Geometry: see drawing. Coordinates: mm, zero at the bounding-box minimum. A direction names the side the tool comes from. Coordinates: 2 decimals unless noted, no trailing zeros. Loops run counter-clockwise (first coordinate to the right, second up) from the corner with the lowest first, then second, coordinate; pieces in that order, holes last. Notation, with made-up numbers: (72, -11) - (121, -11) arc R32 ccw to (121, 15) - close; hole circle Ø1 at (50.25, 5). An arc over 180 degrees is marked (long way). Answer in a Markdown table with one row per item.
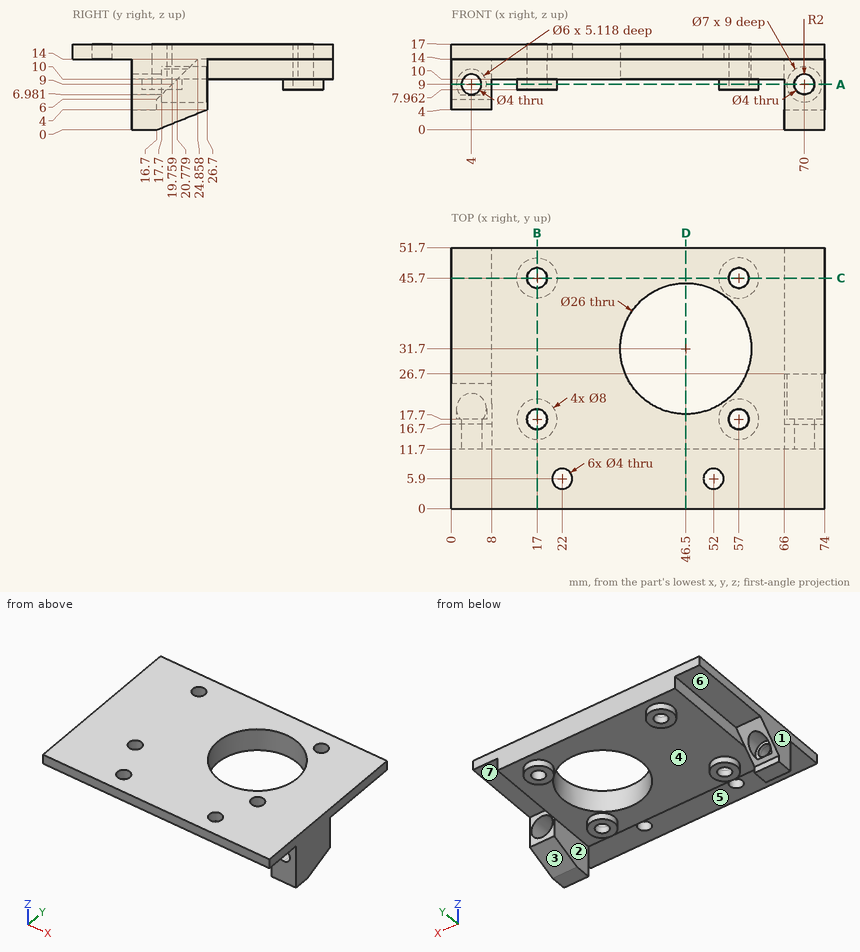
(1) Cut plane D-D on x = 46.5. Output: boundary loops of the cut face in (y, z).
Verdict:
| item | result |
|---|---|
| outline | (0, 14) - (11.7, 14) - (11.7, 10) - (18.7, 10) - (18.7, 17) - (0, 17) - close; (44.7, 10) - (51.7, 10) - (51.7, 17) - (44.7, 17) - close |
(2) Access query for the marked faces 5, 6 and 7. Directions: +Z, -Z, +X, -X, +Y, -Y. A direction counts if a zero-diameter tool reaches every point of the face in a straight line with its end or side. Return the directions, or none.
Verdict:
| item | result |
|---|---|
| face 5 | -Z, +X, -X, -Y |
| face 6 | -Z, -X, +Y |
| face 7 | -Z, +X, +Y |
(3) Cut plane B-B on x = 17. Output: boundary loops of the cut face in (y, z).
Verdict:
| item | result |
|---|---|
| outline | (0, 14) - (11.7, 14) - (11.7, 10) - (13.7, 10) - (13.7, 7.96) - (15.7, 7.96) - (15.7, 17) - (0, 17) - close; (19.7, 7.96) - (21.7, 7.96) - (21.7, 10) - (41.7, 10) - (41.7, 7.96) - (43.7, 7.96) - (43.7, 17) - (19.7, 17) - close; (47.7, 7.96) - (49.7, 7.96) - (49.7, 10) - (51.7, 10) - (51.7, 17) - (47.7, 17) - close |
(4) Pull-direction query (X, two-part tool) for the marked faces 1, 2, 3 and 4; classes: pulls with the +X half, pulls with the -X half, needs draft (parallel to the pull), parting line crosses it, or undercut.
Verdict:
| item | result |
|---|---|
| face 1 | pulls with the -X half |
| face 2 | undercut |
| face 3 | needs draft |
| face 4 | undercut |
(5) First-contact query: pin 1 Ø2 at (y, z) = (27.5, 10) entering from -X; pin 2 Ø3 at (x, z) = (12.5, 11) entering from -Y; pin 3 Ø4.5 at (x, y) = (22, 5.9) entering from -Z. Flat tips, straight axial feed; report the tip coordinate or a pass-through.
Verdict:
| item | result |
|---|---|
| pin 1 | stops at x = 8 |
| pin 2 | stops at y = 11.7 |
| pin 3 | stops at z = 14 |
(6) Cut plane C-C on y = 45.7. Output: boundary loops of the cut face in (x, z).
Verdict:
| item | result |
|---|---|
| outline | (0, 14) - (8, 14) - (8, 10) - (13, 10) - (13, 7.96) - (15, 7.96) - (15, 17) - (0, 17) - close; (19, 7.96) - (21, 7.96) - (21, 10) - (53, 10) - (53, 7.96) - (55, 7.96) - (55, 17) - (19, 17) - close; (59, 7.96) - (61, 7.96) - (61, 10) - (66, 10) - (66, 14) - (74, 14) - (74, 17) - (59, 17) - close |
(7) Ray query, probe 1 along Y at (x, z) = (17, 8.4); probe 2 along Y at (x, z) = (46.5, 15.5); probe 3 along X at (y, z) = (25.25, 9). Return the intervals inside material, ascending.
Verdict:
| item | result |
|---|---|
| probe 1 | y = 13.7 to 15.7, 19.7 to 21.7, 41.7 to 43.7, 47.7 to 49.7 |
| probe 2 | y = 0 to 18.7, 44.7 to 51.7 |
| probe 3 | x = 66 to 66.5, 73.5 to 74 |
(8) Cut plane A-A on z = 9. State how many separate pieces and enclosed holes the cut face has, then the cut area to 3 significant figures.
Verdict:
| item | result |
|---|---|
| separate pieces | 8 |
| enclosed holes | 4 |
| area | 212 mm² |
